```python
from build123d import *

# Parameters (mm, degrees)
SKETCH1_W           = 60
SKETCH1_H           = 40
BOSS_EXTRUDE1_DEPTH = 4
SKETCH2_R           = 3
CUT_EXTRUDE1_DEPTH  = 4
BOSS_EXTRUDE2_START = -2
SKETCH3_R           = 3
SKETCH3_R_2         = 1.5
BOSS_EXTRUDE2_DEPTH = 2


with BuildPart() as part:
    # Sketch1 → Boss-Extrude1 (new body)
    with BuildSketch(Plane(origin=(0, 0, 0), x_dir=(1, 0, 0), z_dir=(0, 1, 0))):
        Rectangle(SKETCH1_W, SKETCH1_H)
    extrude(amount=BOSS_EXTRUDE1_DEPTH)

    # Sketch2 → Cut-Extrude1 (cut)
    with BuildSketch(Plane(origin=(0, 4, 0), x_dir=(1, 0, 0), z_dir=(0, 1, 0))):
        with Locations(Location((0, 0, 0), (0, 0, 270))):
            Circle(SKETCH2_R)
    extrude(amount=-CUT_EXTRUDE1_DEPTH, mode=Mode.SUBTRACT)

    # Sketch3 → Boss-Extrude2 (add)
    with BuildSketch(Plane.XZ.offset(BOSS_EXTRUDE2_START)):
        with Locations(Location((0, 0, 0), (0, 0, 90))):
            Circle(SKETCH3_R)
        with Locations(Location((0, 0, 0), (0, 0, 270))):
            Circle(SKETCH3_R_2, mode=Mode.SUBTRACT)
    extrude(amount=BOSS_EXTRUDE2_DEPTH)


solid = part.part
```
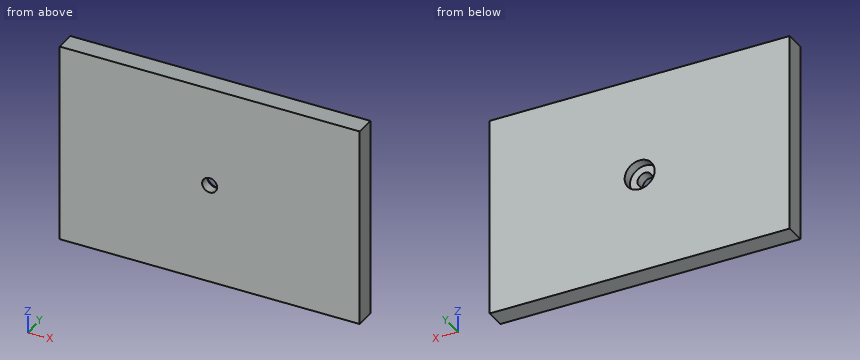
Check sheet for the modelled part. Datum: model origin and axes. Units: mm. Round coordinates to 2 decimals unless told otherwise and drop trailing zeros. Loops run counter-clockwise (first coordinate to the right, second up) from the corner with the lowest first, then second, coordinate; pieces in that order, holes last. Notation, with made-up numbers: (70.5, 84.5) - (85.5, 84.5) arc R26 ccw to (85.5, 99.5) - close; hole circle Ø6 at (19, 16). An arc over 180 degrees is marked (long way). Answer as a JSON object with one key per item and string values. Group by question number.
Q1. Sectioned sample at B-B, the plane x = 0. Enter the section's corners in (y, z), plus the area to 3 significant figures.
Q2. Sectioned sample at A-A, the plane z = 0. Enter the section's corners in (x, y).
Q3. Gauge pin test, flat end, axial feed: P1, Ø6.5, axis at x = 1, z = 0.5, coming from the +Y side. Record the tip position at first contact, or that the pin passes through.
Q4. Scan lines: line 1 along X through (y, z) = (3.45, 0); line 2 along X through (y, z) = (1.3, 0); line 3 along Z through (x, y) = (0, 3.55). Record each from-to range of solid material in increasing order. Write a range as [from, to].
Solution:
{
 "1": {"outline": "(0, -20) - (4, -20) - (4, -3) - (2, -3) - (2, -1.5) - (0, -1.5) - close; (0, 1.5) - (2, 1.5) - (2, 3) - (4, 3) - (4, 20) - (0, 20) - close", "area": "142 mm²"},
 "2": {"outline": "(-30, 0) - (-1.5, 0) - (-1.5, 2) - (-3, 2) - (-3, 4) - (-30, 4) - close; (1.5, 0) - (30, 0) - (30, 4) - (3, 4) - (3, 2) - (1.5, 2) - close"},
 "3": {"P1": "stops at y = 4"},
 "4": {"line 1": "x = [-30, -3], [3, 30]", "line 2": "x = [-30, -1.5], [1.5, 30]", "line 3": "z = [-20, -3], [3, 20]"}
}
